Check sheet for the modelled part. Datum: model origin and axes. Units: mm. Face numbers are marked on the shaded views. A direction names the side the tool comes from. Round coordinates to 2 decimals unless told otherwise and drop trailing zeros. Write each loop counter-clockwise with the first axis right and the second up, starting at its lowest first coordinate (ties: lowest second). Pieces come first, ordered by that corner, then holes. Notation, with made-up numbers: M 51,-37 L 90,-37 A24 cw 90,2 Z; hole C 30,8 d8. An arc over 180 degrees is marked long. Answer in a Markdown table with one row per item.
```python
from build123d import *

# Parameters (mm, degrees)
SKETCH1_W           = 40
SKETCH1_H           = 20
BOSS_EXTRUDE1_DEPTH = 4
SKETCH2_R           = 2.1
CUT_EXTRUDE1_DEPTH  = 4
SKETCH3_W           = 40
SKETCH3_H           = 20
BOSS_EXTRUDE3_DEPTH = 4
SKETCH4_R           = 2.1
CUT_EXTRUDE2_DEPTH  = 4
BOSS_EXTRUDE4_DEPTH = 4
BOSS_EXTRUDE5_DEPTH = 4
CHAMFER1_SIZE       = 1


with BuildPart() as part:
    # Sketch1 → Boss-Extrude1 (new body)
    with BuildSketch(Plane(origin=(0, 0, 0), x_dir=(1, 0, 0), z_dir=(0, 1, 0))):
        with Locations((20, 10)):
            Rectangle(SKETCH1_W, SKETCH1_H)
    extrude(amount=BOSS_EXTRUDE1_DEPTH)

    # Sketch2 → Cut-Extrude1 (cut)
    with BuildSketch(Plane(origin=(0, 4, 0), x_dir=(1, 0, 0), z_dir=(0, 1, 0))):
        with Locations((10, 10)):
            Circle(SKETCH2_R)
        with Locations((30, 10)):
            Circle(SKETCH2_R)
    extrude(amount=-CUT_EXTRUDE1_DEPTH, mode=Mode.SUBTRACT)

    # Sketch3 → Boss-Extrude3 (add)
    with BuildSketch(Plane.XY):
        with Locations((20, 10)):
            Rectangle(SKETCH3_W, SKETCH3_H)
    extrude(amount=-BOSS_EXTRUDE3_DEPTH)

    # Sketch4 → Cut-Extrude2 (cut)
    with BuildSketch(Plane(origin=(0, 0, -4), x_dir=(-1, 0, 0), z_dir=(0, 0, -1))):
        with Locations((-30, 10)):
            Circle(SKETCH4_R)
        with Locations((-10, 10)):
            Circle(SKETCH4_R)
    extrude(amount=-CUT_EXTRUDE2_DEPTH, mode=Mode.SUBTRACT)

    # Sketch5 → Boss-Extrude4 (add)
    with BuildSketch(Plane.ZY):
        Polygon((-20, 4), (-4, 20), (0, 20), (0, 0), (-20, 0), align=None)
    extrude(amount=BOSS_EXTRUDE4_DEPTH)

    # Sketch6 → Boss-Extrude5 (add)
    with BuildSketch(Plane(origin=(40, 0, 0), x_dir=(0, 0, -1), z_dir=(1, 0, 0))):
        Polygon((0, 20), (4, 20), (20, 4), (20, 0), (0, 0), align=None)
    extrude(amount=BOSS_EXTRUDE5_DEPTH)

    # Chamfer1
    chamfer1_edges = [part.edges().sort_by_distance(p)[0] for p in [
        (7.9, 4, -10),
        (27.9, 4, -10),
        (32.1, 10, -4),
        (12.1, 10, -4),
    ]]
    chamfer(chamfer1_edges, length=CHAMFER1_SIZE)


solid = part.part
```
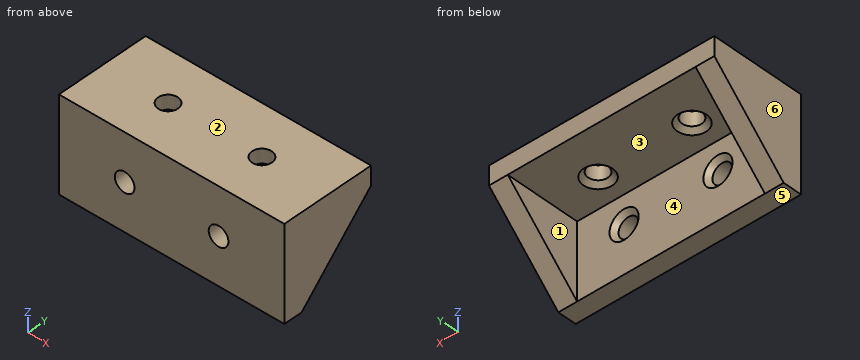
1. Go/stop test with flat-tipped pins: pin 1 (8 mm diameter, centred on x = 13.5, z = -8.5, fed in from +Y); pin 2 (5 mm diameter, centred on x = 12, y = 11, fed in from -Z). Record where each tip stops, or that it passes through.
Found:
| item | result |
|---|---|
| pin 1 | stops at y = 4 |
| pin 2 | stops at z = -4 |
2. Draft check along X on the marked faces 3, 4, 5 and 6. Enter one of: +X half, -X half, draft (parallel to the pull), parting line (faces both ways), or undercut.
Found:
| item | result |
|---|---|
| face 3 | undercut |
| face 4 | undercut |
| face 5 | draft |
| face 6 | -X half |
3. Section check C-C, the plane x = 10. Record the cut outline in (y, z), and give its area (3 significant figures).
Found:
| item | result |
|---|---|
| outline | M 0,-20 L 4,-20 L 4,-13.1 L 3,-12.1 L 0,-12.1 Z; M 0,-7.9 L 3,-7.9 L 4,-6.9 L 4,-4 L 6.9,-4 L 7.9,-3 L 7.9,0 L 0,0 Z; M 12.1,-3 L 13.1,-4 L 20,-4 L 20,0 L 12.1,0 Z |
| area | 108 mm2 |
4. Section check B-B, the plane y = 10. Record the cut outline in (x, z), and give its area (3 significant figures).
Found:
| item | result |
|---|---|
| outline | M -4,-14 L 0,-14 L 0,-4 L 6.9,-4 L 7.9,-3 L 7.9,0 L -4,0 Z; M 12.1,-3 L 13.1,-4 L 26.9,-4 L 27.9,-3 L 27.9,0 L 12.1,0 Z; M 32.1,-3 L 33.1,-4 L 40,-4 L 40,-14 L 44,-14 L 44,0 L 32.1,0 Z |
| area | 236 mm2 |
5. Scan lines: L1, parallel to X at y = 0.85, z = -10; L2, parallel to Z at x = 30, y = 0.9; L3, parallel to X at y = 13, z = -10.5. Record each from-to range of solid material in increasing order.
Found:
| item | result |
|---|---|
| L1 | x = -4 to 7.9, 12.1 to 27.9, 32.1 to 44 |
| L2 | z = -20 to -12.1, -7.9 to 0 |
| L3 | x = -4 to 0, 40 to 44 |
6. Section check D-D, the plane y = 15.75. Record the cut outline in (x, z), and give its area (3 significant figures).
Found:
| item | result |
|---|---|
| outline | M -4,-8.25 L 0,-8.25 L 0,-4 L 40,-4 L 40,-8.25 L 44,-8.25 L 44,0 L -4,0 Z |
| area | 226 mm2 |
7. Section check A-A, the plane z = -10. Record the cut outline in (x, y).
Found:
| item | result |
|---|---|
| outline | M -4,0 L 7.9,0 L 7.9,3 L 6.9,4 L 0,4 L 0,14 L -4,14 Z; M 12.1,0 L 27.9,0 L 27.9,3 L 26.9,4 L 13.1,4 L 12.1,3 Z; M 32.1,0 L 44,0 L 44,14 L 40,14 L 40,4 L 33.1,4 L 32.1,3 Z |
8. Access from +Z, -Z, +X, -X, +Y, -Y to the whole of each face (thin tool, end or side, straight path). Record for the marked faces 1 and 2.
Found:
| item | result |
|---|---|
| face 1 | -Z, +Y |
| face 2 | +Z, +X, -X, +Y, -Y |
